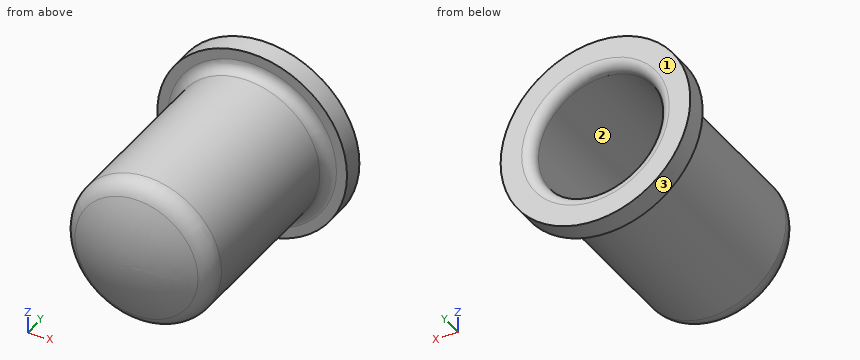
Autodesk Inventor part; units mm, degrees
ref_plane "YZ Plane" through (0, 0, 0) normal (1, 0, 0) x (0, 1, 0)
ref_plane "XZ Plane" through (0, 0, 0) normal (0, 1, 0) x (-1, 0, 0)
ref_plane "XY Plane" through (0, 0, 0) normal (0, 0, 1) x (1, 0, 0)
sketch "Эскиз1" plane through (0, 0, 0) normal (0, 0, 1) x (1, 0, 0)
  line L0 (0, 11) -> (0, -11)
  arc A0 (0, -11) -> (5.8333, -9.7268) centre (0, 3) ccw
  arc A1 (5.8333, -9.7268) -> (7, -7.9087) centre (5, -7.9087) ccw
  line L1 (7, -7.9087) -> (7, 8)
  line L2 (8, 9) -> (9, 9)
  line L3 (9, 9) -> (9, 11)
  line L4 (9, 11) -> (7, 11)
  arc A2 (8, 9) -> (7, 8) centre (8, 8) ccw
  line L5 (6, 10) -> (6, -3)
  arc A3 (0, -9) -> (6, -3) centre (0, -3) ccw
  arc A4 (7, 11) -> (6, 10) centre (7, 10) ccw
  arc A5 (6, -3) -> (6, -3) centre (8, -3) ccw
  line L6 (0, -9) -> (0, -11)
  point P0 (0, 0)
  point P1 (0, 0)
  point P2 (6, -3)
  dimension "d0" = 22
  dimension "d1" = 14
  dimension "d2" = 2
  dimension "d4" = 14
  dimension "d5" = 1
  dimension "d6" = 18
  dimension "d7" = 1
  dimension "d8" = 2
  dimension "d9" = 2
  dimension "d10" = 2
  dimension "d11" = 1
revolve "Вращение1" add sketch "Эскиз1" angle 360 about axis through (0, 11, 0) along (0, -1, 0) picked at (6.6667, -3) contours A3 A5 L1 A1 A0 L0 | L5 A4 L4 L3 L2 A2 L1 A5 | A5 L1
properties part number "79. Предохранитель заднего хода"
The model under review builds one solid part; all positions refer to its coordinate system, in mm. Face numbers are marked on the shaded views. Give positions to 0.01 mm unless a question says otherwise; leave off trailing zeros. Write each loop counter-clockwise with the first axis right and the second up, starting at its lowest first coordinate (ties: lowest second). Pieces come first, ordered by that corner, then holes. Notation, with made-up numbers: (65, -4) - (120, -4) arc R21 cw to (120, 1) - close; hole circle Ø1 at (66, 50). An arc over 180 degrees is marked (long way). Answer in a Markdown table with one row per item. Add a question column.
1. Wall thickness on line 1 along X through (y, z) = (1.5, 0.25); line 2 along Z through (x, y) = (0, 7.5); line 3 along Z through (x, y) = (0.5, 8.5): over which ranges is each line inside the solid? List them lowest first. Write a range as [from, to].
2. We need section B-B on y = -6. Write out the cut boundary in (x, z).
3. We need section A-A on y = 3. Write out the cut boundary in (x, z), then the cut area to 3 significant figures.
4. Insertion check: P1, Ø9.5, axis at x = 0, z = 0, coming from the +Y side; P2, Ø1, axis at x = 0.5, z = -4.5, coming from the -Y side; P3, Ø6, axis at x = 2.5, z = 7, coming from the -Y side. Each pin has a flat end and moves straight along its axis. Give the tip position at first contact, or say it passes through.
5. Draft analysis for pull direction Z (two halves, no side actions). For the marked faces 1, 2 and 3, state which applies: +Z half, -Z half, draft (parallel to the pull), parting line (faces both ways), or undercut.
Ans:
| question | item | result |
|---|---|---|
| 1 | line 1 | x = [-7, -5.99], [5.99, 7] |
| 1 | line 2 | z = [-7, -6], [6, 7] |
| 1 | line 3 | z = [-7.12, -5.98], [5.98, 7.12] |
| 2 | outline | circle Ø14 at (0, 0); hole circle Ø10.39 at (0, 0) |
| 3 | outline | circle Ø14 at (0, 0); hole circle Ø12 at (0, 0) |
| 3 | area | 40.8 mm^2 |
| 4 | P1 | stops at y = -6.67 |
| 4 | P2 | stops at y = -10.41 |
| 4 | P3 | stops at y = -10.28 |
| 5 | face 1 | draft |
| 5 | face 2 | undercut |
| 5 | face 3 | parting line |
